from build123d import *

# Parameters (mm, degrees)
SKETCH1_W           = 200
SKETCH1_H           = 350
SKETCH1_R           = 5
BOSS_EXTRUDE1_DEPTH = 6
FILLET1_R           = 10
SKETCH2_W           = 12
SKETCH2_H           = 50
SKETCH2_W_2         = 54
SKETCH2_H_2         = 80
SKETCH2_W_3         = 12.25
SKETCH2_H_3         = 21
CUT_EXTRUDE1_DEPTH  = 7


with BuildPart() as part:
    # Sketch1 → Boss-Extrude1 (new body)
    with BuildSketch(Plane.XY):
        Rectangle(SKETCH1_W, SKETCH1_H)
        with Locations((-57.588571429, 100.78)):
            Circle(SKETCH1_R, mode=Mode.SUBTRACT)
        with Locations((57.588571429, 100.78)):
            Circle(SKETCH1_R, mode=Mode.SUBTRACT)
        with Locations((57.588571429, -100.78)):
            Circle(SKETCH1_R, mode=Mode.SUBTRACT)
        with Locations((-57.588571429, -100.78)):
            Circle(SKETCH1_R, mode=Mode.SUBTRACT)
    extrude(amount=BOSS_EXTRUDE1_DEPTH)

    # Fillet1
    fillet1_edges = [part.edges().sort_by_distance(p)[0] for p in [
        (100, -175, 3),
        (-100, -175, 3),
        (-100, 175, 3),
        (100, 175, 3),
    ]]
    fillet(fillet1_edges, radius=FILLET1_R)

    # Sketch2 → Cut-Extrude1 (cut, through all)
    with BuildSketch(Plane.XY.offset(6)):
        Polygon((10.001494726, 113), (17.551494726, 113), (17.551494726, 17), (-64.448505274, 17), (-64.448505274, 113), (0.001494726, 113), (0.001494726, 145.880160171), (10.001494726, 145.880160171), align=None)
        with Locations((-84, 115)):
            Rectangle(SKETCH2_W, SKETCH2_H)
        with Locations((-84, -125)):
            Rectangle(SKETCH2_W, SKETCH2_H)
        with Locations((84, -125)):
            Rectangle(SKETCH2_W, SKETCH2_H)
        with Locations((84, 115)):
            Rectangle(SKETCH2_W, SKETCH2_H)
        with Locations((-74, -35)):
            Rectangle(SKETCH2_W_2, SKETCH2_H_2)
        with Locations((0, -149)):
            Rectangle(SKETCH2_W_3, SKETCH2_H_3)
    extrude(amount=-CUT_EXTRUDE1_DEPTH, mode=Mode.SUBTRACT)


solid = part.part
Model file for the job. Use its own axes, mm. Round coordinates to 2 decimals unless told otherwise and drop trailing zeros. Order: outer loops, then holes, each group sorted by start corner. A loop starts at its lowest first (then second) coordinate and runs counter-clockwise, first axis right, second up. Notation, with made-up numbers: M -6.5,77 L 32.5,77 A29 cw 32.5,110 Z; hole C 31.25,52 d4. An arc over 180 degrees is marked long. Write each question's results on one line, items separated by ' | '. Start each with the question number.
(1) Saw through at B-B, the plane y = 44.5. Give the cut face in (x, z), then the cut area to 3 significant figures.
(2) Probe probe 1 along X at (y, z) = (-146, 2) (3 decimals); probe 2 along X at (y, z) = (-119.5, 0.45); probe 3 along X at (y, z) = (129, 2.3). List the from-to ranges inside material, lowest first. Write a range as from..to.
(3) Drop a flat-ended pin along its axis: pin 1 (5 mm diameter, centred on x = -61.5, y = 75, fed in from +Z). Give the stop position or say it passes through.
(4) Two-plate mould, pull along Y, no slides. Class faces 1 (the face through (-54.901, -96.564, 2.958)), 2 (the face through (-1, 2, 0)), 3 (the face through (56.5, 95.9, 3)), 4 (the face through (-97.15, 171.99, 3.04)): pulls with the +Y half, pulls with the -Y half, needs draft (parallel to the pull), parting line crosses it, or undercut.
(5) Saw through at C-C, the plane x = -86. Give the cut face in (y, z).
(6) Saw through at A-A, the plane y = 120.5. Give the cut face in (x, z), then the cut area to 3 significant figures.
(7) Saw through at D-D, the plane x = -42. Give the cut face in (y, z), then the cut area to 3 significant figures.
Established:
1) outline: M -100,0 L -64.45,0 L -64.45,6 L -100,6 Z; M 17.55,0 L 100,0 L 100,6 L 17.55,6 Z | area: 708 mm^2
2) probe 1: x = -100..-90, -78..-6.125, 6.125..78, 90..100 | probe 2: x = -100..-90, -78..78, 90..100 | probe 3: x = -100..-90, -78..0, 10..78, 90..100
3) pin 1: passes through
4) face 1: undercut | face 2: needs draft | face 3: undercut | face 4: pulls with the +Y half
5) outline: M -175,0 L -150,0 L -150,6 L -175,6 Z; M -100,0 L -75,0 L -75,6 L -100,6 Z; M 5,0 L 90,0 L 90,6 L 5,6 Z; M 140,0 L 175,0 L 175,6 L 140,6 Z
6) outline: M -100,0 L -90,0 L -90,6 L -100,6 Z; M -78,0 L 0,0 L 0,6 L -78,6 Z; M 10,0 L 78,0 L 78,6 L 10,6 Z; M 90,0 L 100,0 L 100,6 L 90,6 Z | area: 996 mm^2
7) outline: M -175,0 L 17,0 L 17,6 L -175,6 Z; M 113,0 L 175,0 L 175,6 L 113,6 Z | area: 1,520 mm^2
